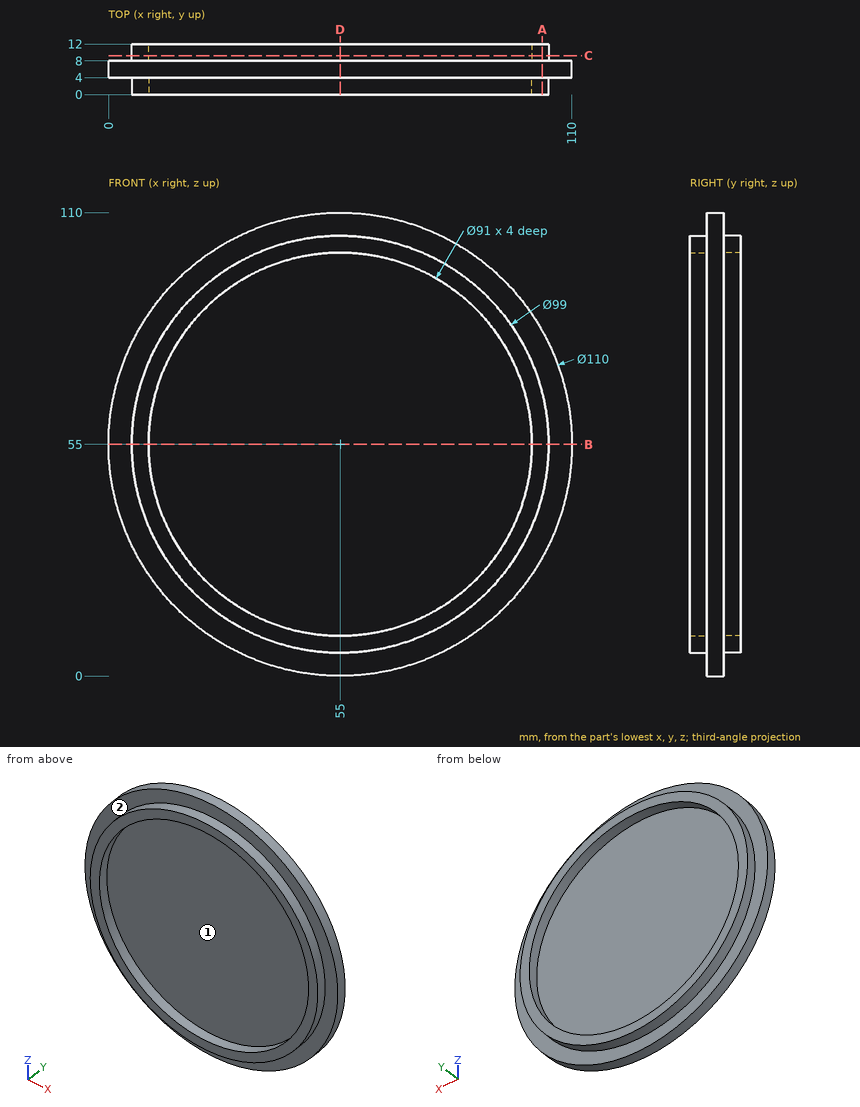
Could you check a few things on this drawing? It's one solid part, dimensions in mm from its lowest x, y, z. Round coordinates to 2 decimals unless told otherwise and drop trailing zeros. Order: outer loops, then holes, each group sorted by start corner. A loop starts at its lowest first (then second) coordinate and runs counter-clockwise, first axis right, second up.
(1) If we mould it in two halves opening along X, with no side actions, what happens to the marked faces 1 and 2? For each: released by +X, released by -X, zero draft, split by the parting line, or undercut.
Response values:
face 1: undercut
face 2: zero draft
(2) I'm going to push flat-ended pins straight in: pin 1 (4 mm diameter, centred on y = 7.5, z = 11.5, fed in from -X); pin 2 (1 mm diameter, centred on x = 38, z = 59.5, fed in from -Y); pin 3 (6 mm diameter, centred on y = 3.5, z = 82.5, fed in from -X). Where does each tip first touch, or does it pass through?
Response values:
pin 1: stops at x = 18.91
pin 2: stops at y = 4
pin 3: stops at x = 5.78
(3) Please list where these lines run through material, in increasing order: line 1 along Z through (x, y) = (55, 9.1); line 2 along Y through (x, z) = (36, 18).
Response values:
line 1: z = 5.5 to 9.5, 100.5 to 104.5
line 2: y = 4 to 8
(4) Imagine slicing it at C-C (y = 9.25). Write out the boundary of the cut face in (x, z).
Response values:
outline: circle Ø99 at (55, 55); hole circle Ø91 at (55, 55)
(5) Imagine slicing it at A-A (x = 103). Write out the boundary of the cut face in (y, z).
Response values:
outline: (0, 42.91) - (4, 42.91) - (4, 28.15) - (8, 28.15) - (8, 42.91) - (12, 42.91) - (12, 67.09) - (8, 67.09) - (8, 81.85) - (4, 81.85) - (4, 67.09) - (0, 67.09) - close
(6) Imagine slicing it at D-D (x = 55). Write out the boundary of the cut face in (y, z), plus the area to 3 significant figures.
Response values:
outline: (0, 5.5) - (4, 5.5) - (4, 0) - (8, 0) - (8, 5.5) - (12, 5.5) - (12, 9.5) - (8, 9.5) - (8, 100.5) - (12, 100.5) - (12, 104.5) - (8, 104.5) - (8, 110) - (4, 110) - (4, 104.5) - (0, 104.5) - (0, 100.5) - (4, 100.5) - (4, 9.5) - (0, 9.5) - close
area: 504 mm2
(7) Imagine slicing it at B-B (z = 55). Write out the boundary of the cut face in (x, y).
Response values:
outline: (0, 4) - (5.5, 4) - (5.5, 0) - (9.5, 0) - (9.5, 4) - (100.5, 4) - (100.5, 0) - (104.5, 0) - (104.5, 4) - (110, 4) - (110, 8) - (104.5, 8) - (104.5, 12) - (100.5, 12) - (100.5, 8) - (9.5, 8) - (9.5, 12) - (5.5, 12) - (5.5, 8) - (0, 8) - close
